The listing builds one solid part. Answer for the finished solid, in the listing's coordinates (mm). Face numbers are marked on the shaded views. Give positions to 0.01 mm unless a question says otherwise; leave off trailing zeros. Loops run counter-clockwise (first coordinate to the right, second up) from the corner with the lowest first, then second, coordinate; pieces in that order, holes last.
Item 1: Each of these flat-tipped pins is pushed along its axis until it touches: pin 1 Ø1.8 at (x, z) = (0, -5) entering from -Y; pin 2 Ø3.5 at (x, z) = (-5, 5) entering from -Y. Where does it stop, or does it pass through?
Item 2: The mould has two halves that part along X. Classify the marked faces 1, 2, 3 and 4: pulls with the +X half, pulls with the -X half, needs draft (parallel to the pull), parting line crosses it, or undercut.
Item 3: Section C-C, the plane x = 1 is taken. Give the vertices of the cut face in (y, z), and give its area (3 significant figures).
Item 4: Consider line 1 along Z through (x, y) = (0, 1.45); line 2 along Z through (x, y) = (11, 2.9). Determine where each line is inside the solid, lowest interval first.
Item 5: Section A-A, the plane z = 0 is taken. Give the number of separate pieces and of enclosed holes in the cut face, and give its area (3 significant figures).
Item 6: Section D-D, the plane x = 5 is taken. Give the vertices of the cut face in (y, z), and give its area (3 significant figures).
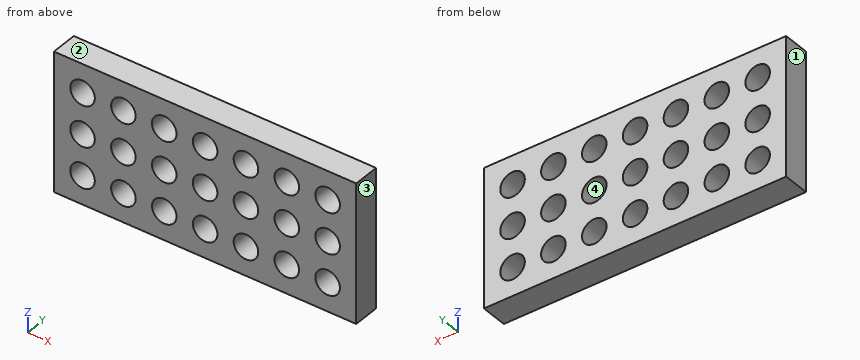
from build123d import *

# Parameters (mm, degrees)
SKETCH1_W           = 37
SKETCH1_H           = 17
SKETCH1_R           = 1.5025
BOSS_EXTRUDE1_DEPTH = 3.25


with BuildPart() as part:
    # Sketch1 → Boss-Extrude1 (new body)
    with BuildSketch(Plane(origin=(0, 0, 0), x_dir=(1, 0, 0), z_dir=(0, 1, 0))):
        Rectangle(SKETCH1_W, SKETCH1_H)
        with Locations((-15, -5)):
            Circle(SKETCH1_R, mode=Mode.SUBTRACT)
        with Locations((-10, -5)):
            Circle(SKETCH1_R, mode=Mode.SUBTRACT)
        with Locations((-5, -5)):
            Circle(SKETCH1_R, mode=Mode.SUBTRACT)
        with Locations((0, -5)):
            Circle(SKETCH1_R, mode=Mode.SUBTRACT)
        with Locations((5, -5)):
            Circle(SKETCH1_R, mode=Mode.SUBTRACT)
        with Locations((10, -5)):
            Circle(SKETCH1_R, mode=Mode.SUBTRACT)
        with Locations((15, -5)):
            Circle(SKETCH1_R, mode=Mode.SUBTRACT)
        with Locations((-10, 0)):
            Circle(SKETCH1_R, mode=Mode.SUBTRACT)
        with Locations((-5, 0)):
            Circle(SKETCH1_R, mode=Mode.SUBTRACT)
        Circle(SKETCH1_R, mode=Mode.SUBTRACT)
        with Locations((5, 0)):
            Circle(SKETCH1_R, mode=Mode.SUBTRACT)
        with Locations((10, 0)):
            Circle(SKETCH1_R, mode=Mode.SUBTRACT)
        with Locations((15, 0)):
            Circle(SKETCH1_R, mode=Mode.SUBTRACT)
        with Locations((-10, 5)):
            Circle(SKETCH1_R, mode=Mode.SUBTRACT)
        with Locations((-5, 5)):
            Circle(SKETCH1_R, mode=Mode.SUBTRACT)
        with Locations((0, 5)):
            Circle(SKETCH1_R, mode=Mode.SUBTRACT)
        with Locations((5, 5)):
            Circle(SKETCH1_R, mode=Mode.SUBTRACT)
        with Locations((10, 5)):
            Circle(SKETCH1_R, mode=Mode.SUBTRACT)
        with Locations((15, 5)):
            Circle(SKETCH1_R, mode=Mode.SUBTRACT)
        with Locations((-15, 0)):
            Circle(SKETCH1_R, mode=Mode.SUBTRACT)
        with Locations((-15, 5)):
            Circle(SKETCH1_R, mode=Mode.SUBTRACT)
    extrude(amount=BOSS_EXTRUDE1_DEPTH)


solid = part.part
Worked answers:
1. pin 1: passes through
1. pin 2: stops at y = 0
2. face 1: pulls with the -X half
2. face 2: needs draft
2. face 3: pulls with the +X half
2. face 4: undercut
3. outline: (0, -8.5) - (3.25, -8.5) - (3.25, -6.12) - (0, -6.12) - close; (0, -3.88) - (3.25, -3.88) - (3.25, -1.12) - (0, -1.12) - close; (0, 1.12) - (3.25, 1.12) - (3.25, 3.88) - (0, 3.88) - close; (0, 6.12) - (3.25, 6.12) - (3.25, 8.5) - (0, 8.5) - close
3. area: 33.4 mm2
4. line 1: z = -8.5 to -6.5, -3.5 to -1.5, 1.5 to 3.5, 6.5 to 8.5
4. line 2: z = -8.5 to -6.12, -3.88 to -1.12, 1.12 to 3.88, 6.12 to 8.5
5. separate pieces: 8
5. enclosed holes: 0
5. area: 51.9 mm2
6. outline: (0, -8.5) - (3.25, -8.5) - (3.25, -6.5) - (0, -6.5) - close; (0, -3.5) - (3.25, -3.5) - (3.25, -1.5) - (0, -1.5) - close; (0, 1.5) - (3.25, 1.5) - (3.25, 3.5) - (0, 3.5) - close; (0, 6.5) - (3.25, 6.5) - (3.25, 8.5) - (0, 8.5) - close
6. area: 26.0 mm2
